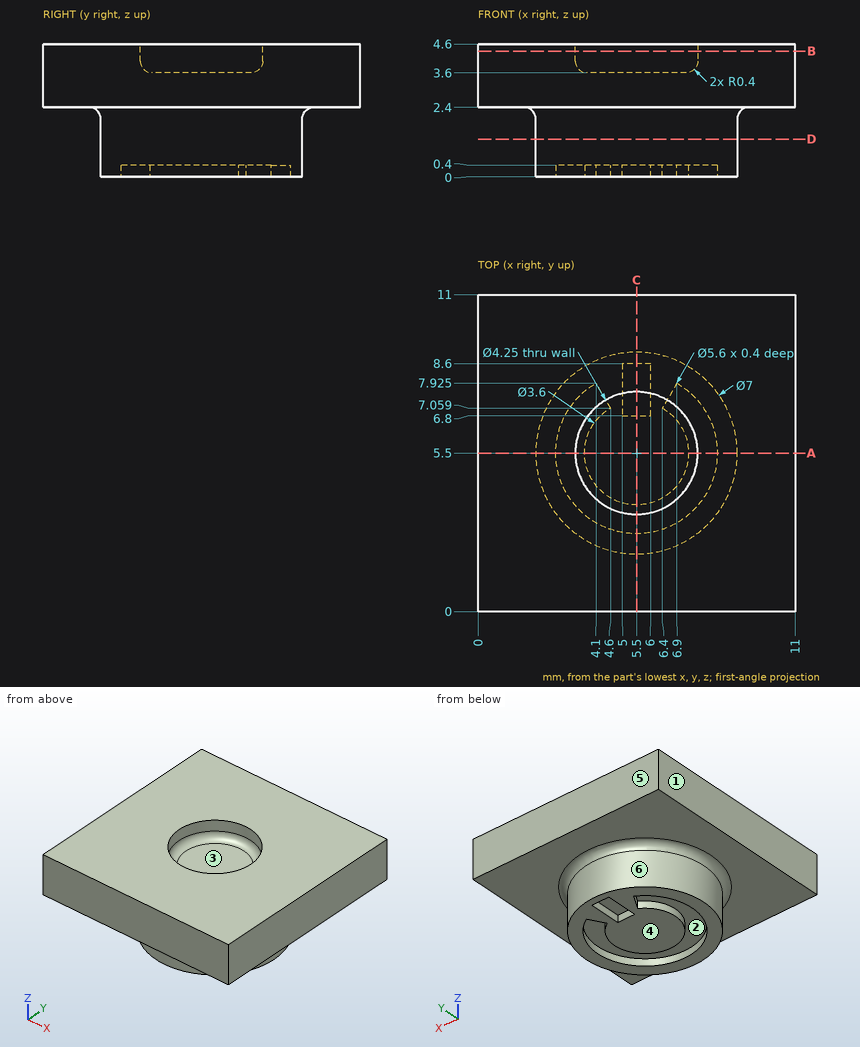
Verification items for this drawing (mm, ordinates from the low corner). A direction names the side the tool comes from. Coordinates: 2 decimals unless noted, no trailing zeros. Order: outer loops, then holes, each group sorted by start corner. A loop starts at its lowest first (then second) coordinate and runs counter-clockwise, first axis right, second up. Notation, with made-up numbers: (66.25, -7.75) - (86.25, -7.75) arc R35 ccw to (86.25, 30.25) - close; hole circle Ø8 at (-31.75, 49.25). An arc over 180 degrees is marked (long way). Answer as a JSON object with one key per item and string values. Group by question number.
Item 1: Sectioned sample at A-A, the plane y = 5.5. Record the cut outline in (x, z) (3 decimals), and give its area (3 significant figures).
Item 2: Scan lines: probe 1 along Y at (x, z) = (5.5, 0.3); probe 2 along Y at (x, z) = (5.5, 4.35) (3 decimals); probe 3 along Z at (x, y) = (6, 3). Record each from-to range of solid material in increasing order.
Item 3: Sectioned sample at D-D, the plane z = 1.3. Record the cut outline in (x, y), and give its area (3 significant figures).
Item 4: Sectioned sample at C-C, the plane x = 5.5. Record the cut outline in (y, z) (3 decimals).
Item 5: Draft check along X on the marked faces 1, 2, 3 and 4. Enter one of: +X half, -X half, draft (parallel to the pull), parting line (faces both ways), or undercut.
Item 6: Tool access check on the marked faces 5 and 6. Record the directions out of +Z, -Z, +X, -X, +Y, -Y that give a thin tool (end or side, any length) a straight path to the whole face; none if there is none.
Item 7: Sectioned sample at B-B, the plane z = 4.35. Record the cut outline in (x, y) (3 decimals).
Item 8: Depth check by flat-ended pin: pin 1 Ø2 at (x, z) = (8, 1) entering from -Y; pin 2 Ø1 at (x, y) = (5, 6.5) entering from +Z; pin 3 Ø4 at (x, y) = (5.5, 5.5) entering from +Z. Enter the tip coordinate at first touch or a pass-through.
Resolved:
{
 "1": {"outline": "(0, 2.4) - (1.6, 2.4) arc R0.4 cw to (2, 2) - (2, 0) - (2.7, 0) - (2.7, 0.4) - (3.7, 0.4) - (3.7, 0) - (7.3, 0) - (7.3, 0.4) - (8.3, 0.4) - (8.3, 0) - (9, 0) - (9, 2) arc R0.4 cw to (9.4, 2.4) - (11, 2.4) - (11, 4.6) - (7.625, 4.6) - (7.625, 4) arc R0.4 cw to (7.225, 3.6) - (3.775, 3.6) arc R0.4 cw to (3.375, 4) - (3.375, 4.6) - (0, 4.6) - close", "area": "36.1 mm^2"},
 "2": {"probe 1": "2 to 2.7, 3.7 to 6.8, 8.6 to 9", "probe 2": "0 to 3.375, 7.625 to 11", "probe 3": "0.4 to 4.6"},
 "3": {"outline": "circle Ø7 at (5.5, 5.5)", "area": "38.5 mm^2"},
 "4": {"outline": "(0, 2.4) - (1.6, 2.4) arc R0.4 cw to (2, 2) - (2, 0) - (2.7, 0) - (2.7, 0.4) - (3.7, 0.4) - (3.7, 0) - (6.8, 0) - (6.8, 0.4) - (8.6, 0.4) - (8.6, 0) - (9, 0) - (9, 2) arc R0.4 cw to (9.4, 2.4) - (11, 2.4) - (11, 4.6) - (7.625, 4.6) - (7.625, 4) arc R0.4 cw to (7.225, 3.6) - (3.775, 3.6) arc R0.4 cw to (3.375, 4) - (3.375, 4.6) - (0, 4.6) - close"},
 "5": {"face 1": "-X half", "face 2": "undercut", "face 3": "undercut", "face 4": "draft"},
 "6": {"face 5": "+Z, -Z, +X, -X, +Y", "face 6": "-Z"},
 "7": {"outline": "(0, 0) - (11, 0) - (11, 11) - (0, 11) - close; hole circle Ø4.25 at (5.5, 5.5)"},
 "8": {"pin 1": "y = 2.34", "pin 2": "z = 3.6", "pin 3": "z = 3.71"}
}
